Geometry check sheet. Reference: the model listing, model coordinates, mm. A direction names the side the tool comes from. Give positions to 0.01 mm unless a question says otherwise; leave off trailing zeros. Loops run counter-clockwise (first coordinate to the right, second up) from the corner with the lowest first, then second, coordinate; pieces in that order, holes last. Notation, with made-up numbers: (-37, 41) - (17, 41) arc R14 ccw to (17, 47) - close; hole circle Ø9 at (61, -16). An arc over 180 degrees is marked (long way). Use a Markdown table: item, result. Add a question column.
1. Cross-section at C-C on x = 290.5. Enter the section's corners in (y, z) (1 decimal), and give its area (3 significant figures).
2. Draft check along Z on faces 4 (the cylindrical face through (172.18, 3.34, -10.6)), 5 (the cylindrical face through (130.131, -15.497, 3.441)), 6 (the flat face through (0, -11.4, 0.2)). Enter one of: pulls with the +Z half, pulls with the -Z half, needs draft (parallel to the pull), parting line crosses it, or undercut.
3. Set-up check for faces 1 (the cylindrical face through (10, 17, -4)), 2 (the flat face through (133.35, 8.31, 11.83)), 3 (the flat face through (127, 8.31, 11.83)): record each of +Z, -Z, +X, -X, +Y, -Y from which the full face is reachable in a straight line by a thin tool's end or side.
4. Depth check by flat-ended pin: P1, Ø3, axis at y = 0.5, z = -8.5, coming from the -X side; P2, Ø1.5, axis at x = 39.5, y = -12, coming from the -Z side; P3, Ø5, axis at x = 87, y = -11, coming from the -Z side; P4, Ø8, axis at x = 195, z = 1.5, coming from the -Y side. Enter the tip coordinate at first touch or a pass-through.
5. Material ranges on L1, parallel to Y at x = 254, z = 0; L2, parallel to Y at x = 166, z = -4.5; L3, parallel to Z at x = 84.5, y = -5, recorded low to high.
from build123d import *

# Parameters (mm, degrees)
SKETCH1_R           = 14.2875
SKETCH1_R_2         = 11.1125
BOSS_EXTRUDE1_DEPTH = 349.25
SKETCH2_R           = 15.875
SKETCH2_R_2         = 12.674707898
BOSS_EXTRUDE2_DEPTH = 6.35


with BuildPart() as part:
    # Sketch1 → Boss-Extrude1 (new body)
    with BuildSketch(Plane(origin=(0, 0, 0), x_dir=(0, 0, -1), z_dir=(1, 0, 0))):
        Circle(SKETCH1_R)
        Circle(SKETCH1_R_2, mode=Mode.SUBTRACT)
    extrude(amount=BOSS_EXTRUDE1_DEPTH)

    # Sketch2 → Boss-Extrude2 (add)
    with BuildSketch(Plane(origin=(127, 0, 0), x_dir=(0, 0, -1), z_dir=(1, 0, 0))):
        Circle(SKETCH2_R)
        Circle(SKETCH2_R_2, mode=Mode.SUBTRACT)
    extrude(amount=BOSS_EXTRUDE2_DEPTH)

    # Sketch3 → Revolve1 (revolve)
    with BuildSketch(Plane.XY, mode=Mode.PRIVATE) as revolve1_sk:
        Polygon((23.8125, 12.531653429), (0, 12.531653429), (0, 17.4625), (19.05, 17.4625), (23.8125, 14.2875), align=None)
    revolve(revolve1_sk.sketch.rotate(Axis((0, 0, 0), (1, 0, 0)), 90), axis=Axis((0, 0, 0), (1, 0, 0)))


solid = part.part
Values found:
| question | item | result |
|---|---|---|
| 1 | outline | circle Ø28.6 at (0, 0); hole circle Ø22.2 at (0, 0) |
| 1 | area | 253 mm2 |
| 2 | face 4 | undercut |
| 2 | face 5 | parting line crosses it |
| 2 | face 6 | needs draft |
| 3 | face 1 | +X, -X |
| 3 | face 2 | +X |
| 3 | face 3 | none |
| 4 | P1 | passes through |
| 4 | P2 | stops at z = -8.81 |
| 4 | P3 | stops at z = -11.48 |
| 4 | P4 | stops at y = -14.29 |
| 5 | L1 | y = -14.29 to -11.11, 11.11 to 14.29 |
| 5 | L2 | y = -13.56 to -10.16, 10.16 to 13.56 |
| 5 | L3 | z = -13.38 to -9.92, 9.92 to 13.38 |
